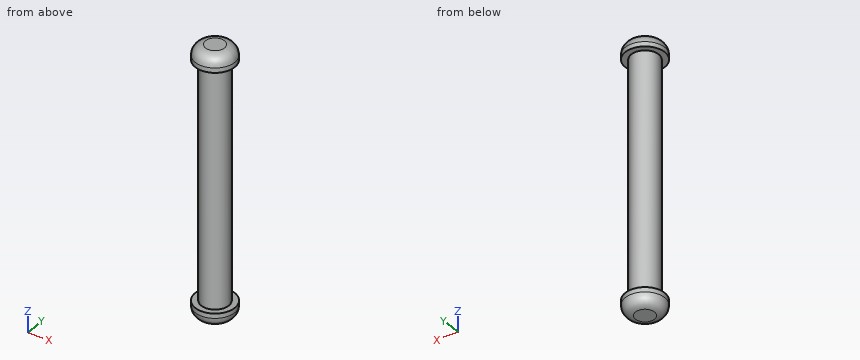
Autodesk Inventor part; units mm, degrees
ref_plane "YZ Plane" through (0, 0, 0) normal (1, 0, 0) x (0, 1, 0)
ref_plane "XZ Plane" through (0, 0, 0) normal (0, 1, 0) x (-1, 0, 0)
ref_plane "XY Plane" through (0, 0, 0) normal (0, 0, 1) x (1, 0, 0)
sketch "Sketch1" plane through (0, 0, 0) normal (0, 0, 1) x (1, 0, 0)
  circle A0 centre (0, 0) radius 4.445
  dimension "d0" = 8.89
extrude "Extrusion1" add sketch "Sketch1" along normal mid plane 76.2
sketch "Sketch2" plane through (0, 0, 38.1) normal (0, 0, 1) x (1, 0, 0)
  circle A0 centre (0, 0) radius 6.35
  dimension "d3" = 12.7
extrude "Extrusion2" add sketch "Sketch2" along normal blind 4.826
fillet "Fillet1" radius 3.302 1 edges at (-6.35, 0, 42.926)
mirror "Mirror1" about plane through (0, 0, 0) normal (0, 0, 1) of "Extrusion2", "Fillet1"
properties part number "3 Inch Pin"
For this review, take the finished solid that the model builds, in its own axes (mm). Round coordinates to 2 decimals unless told otherwise and drop trailing zeros. Write each loop counter-clockwise with the first axis right and the second up, starting at its lowest first coordinate (ties: lowest second). Pieces come first, ordered by that corner, then holes. Notation, with made-up numbers: (25, -26) - (41, -26) arc R15 cw to (41, 2) - close; hole circle Ø5 at (-35, 51). An arc over 180 degrees is marked (long way). Answer as a JSON object with one key per item and string values.
1. To check wall thickness, follow line 1 along Y through (x, z) = (-3.25, 21.5); line 2 along Y through (x, z) = (-0.25, -28); line 3 along Z through (x, y) = (-2, -2.5). State the ranges of each line that lie inside material, in increasing order.
Response values:
{"line 1": "y = -3.03 to 3.03", "line 2": "y = -4.44 to 4.44", "line 3": "z = -42.92 to 42.92"}
2. We need section A-A on z = 15.5. Give the boundary of the cut face in (x, y) (3 decimals), then the cut area to 3 significant figures.
Response values:
{"outline": "circle Ø8.89 at (0, 0)", "area": "62.1 mm2"}
3. For pin 1 Ø4 at (y, z) = (-4.5, -4.5) entering from -X; pin 2 Ø5 at (x, z) = (3.5, 31) entering from +Y; pin 3 Ø5 at (x, y) = (-3.5, -0.5) entering from -Z; pin 4 Ø5 at (x, z) = (5, 5.5) entering from +Y, all flat-tipped, find the tip position at first contact; note any pin that passes through.
Response values:
{"pin 1": "stops at x = -3.68", "pin 2": "stops at y = 4.33", "pin 3": "stops at z = -42.93", "pin 4": "stops at y = 3.68"}
